```python
from build123d import *

# Parameters (mm, degrees)
SALIENTE_EXTRUIR1_DEPTH = 1.25


with BuildPart() as part:
    # Croquis1 → Revolución1 (revolve)
    with BuildSketch(Plane.XY, mode=Mode.PRIVATE) as revoluci_n1_sk:
        Polygon((0, 0), (37, 0), (37, 3), (31, 3), (31, 3.75), (2, 3.75), (2, 8), (0, 8), align=None)
    revolve(revoluci_n1_sk.sketch.rotate(Axis((0, 0, 0), (1, 0, 0)), 90), axis=Axis((0, 0, 0), (1, 0, 0)))

    # Croquis2 → Saliente-Extruir1 (add, symmetric)
    with BuildSketch(Plane.XY):
        Polygon((2, 5.164213562), (3.414213562, 3.75), (5.426219931, 1.737993631), (0.712521071, 1.737993631), (0.712521071, 6.451692492), align=None)
    extrude(amount=SALIENTE_EXTRUIR1_DEPTH, both=True)


solid = part.part
```
Work out the finished part from the listing and answer in its coordinate system (mm). A direction names the side the tool comes from. Give positions to 0.01 mm unless a question says otherwise; leave off trailing zeros. Loops run counter-clockwise (first coordinate to the right, second up) from the corner with the lowest first, then second, coordinate; pieces in that order, holes last. Notation, with made-up numbers: M 5,-26.5 L 30,-26.5 A16 ccw 30,-12.5 Z; hole C 81,73.25 d8. An arc over 180 degrees is marked long. One line per item, written item: value. Start each with the question number.
1. Find section D-D (y = 4.5). Give the vertices of the cut face in (x, z), and give its area (3 significant figures).
2. Find section B-B (z = 0). Give the vertices of the cut face in (x, y).
3. Find section A-A (y = 0). Give the vertices of the cut face in (x, z), and give its area (4 significant figures).
4. Find section C-C (x = 17). Give the vertices of the cut face in (y, z), and give its area (3 significant figures).
5. Which of the six approach directions +Z, -Z, +X, -X, +Y, -Y give full straight-line access (tool end or side, diameter ignored) to faces 1 (the face through (2.5, 4, -1.25)), 2 (the face through (2.5, 4, 1.25)), 3 (the face through (16.3, -3.16, 2.02))?
6. Each of these flat-tipped pins is pushed along its axis until it touches: P1, Ø8, axis at x = 20, z = -5, coming from the -Y side; P2, Ø2, axis at x = 24.5, y = 0, coming from the -Z side; P3, Ø1, axis at x = 19.5, y = -3.5, coming from the -Z side. Where does it stop, or does it pass through?
7. Find the intervals of material crossed by probe 1 along X at (y, z) = (-1.5, 3.75); probe 2 along X at (y, z) = (-1.75, 2.5); probe 3 along Z at (x, y) = (30, -1), in increasing order.
Reported:
1. outline: M 0,-6.61 L 2,-6.61 L 2,-1.25 L 2.66,-1.25 L 2.66,1.25 L 2,1.25 L 2,6.61 L 0,6.61 Z
1. area: 28.1 mm²
2. outline: M 0,-8 L 2,-8 L 2,-3.75 L 31,-3.75 L 31,-3 L 37,-3 L 37,3 L 31,3 L 31,3.75 L 3.41,3.75 L 2,5.16 L 2,8 L 0,8 Z
3. outline: M 0,-8 L 2,-8 L 2,-3.75 L 31,-3.75 L 31,-3 L 37,-3 L 37,3 L 31,3 L 31,3.75 L 2,3.75 L 2,8 L 0,8 Z
3. area: 285.5 mm²
4. outline: C 0,0 d7.5
4. area: 44.2 mm²
5. face 1: -Z, +X, +Y
5. face 2: +Z, +X, +Y
5. face 3: +X
6. P1: stops at y = -3.61
6. P2: stops at z = -3.75
6. P3: stops at z = -2.25
7. probe 1: x = 0 to 2
7. probe 2: x = 0 to 31
7. probe 3: z = -3.61 to 3.61
